Here's how the part is built. I have some questions about the finished solid (model axes, mm). Face numbers are marked on the shaded views. Round coordinates to 2 decimals unless told otherwise and drop trailing zeros. Loops run counter-clockwise (first coordinate to the right, second up) from the corner with the lowest first, then second, coordinate; pieces in that order, holes last. Notation, with made-up numbers: M 86,-21 L 104,-21 A14 ccw 104,4 Z; hole C 89.25,-8.75 d4. An arc over 180 degrees is marked long. Put each result on its own line as item: value. Start each with the question number.
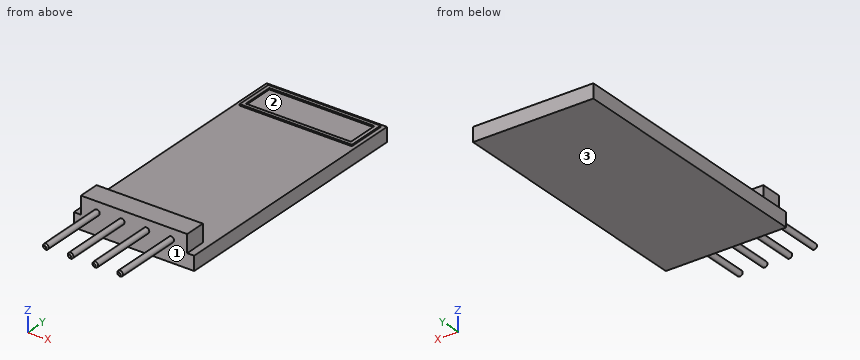
```python
from build123d import *

# Parameters (mm, degrees)
F0_W     = 17
F0_H     = 37
F1_DEPTH = 1
F2_W     = 15
F2_H     = 3
F3_DEPTH = 2.5
F4_R     = 0.4
F5_DEPTH = 10
F6_SIZE  = 0.2
F7_W     = 15.8485004902
F7_H     = 5.5060135201
F7_W_2   = 14.8485004902
F7_H_2   = 4.5060135201
F8_DEPTH = 0.2


with BuildPart() as f1:
    # F0 (on Top) → F1 (new body, symmetric)
    with BuildSketch(Plane.XY):
        Rectangle(F0_W, F0_H)
    extrude(amount=F1_DEPTH, both=True)

    # F2 (on face) → F3 (join)
    with BuildSketch(Plane.XY.offset(1)):
        with Locations((0, -17)):
            Rectangle(F2_W, F2_H)
    extrude(amount=F3_DEPTH)

    # F4 (on face) → F5 (join)
    with BuildSketch(Plane.XZ.offset(18.5)):
        with Locations((-5.25, 2.0477680955)):
            Circle(F4_R)
        with Locations((-1.75, 2.0477680955)):
            Circle(F4_R)
        with Locations((1.75, 2.0477680955)):
            Circle(F4_R)
        with Locations((5.25, 2.0477680955)):
            Circle(F4_R)
    extrude(amount=F5_DEPTH)

    # F6
    f6_edges = [f1.edges().sort_by_distance(p)[0] for p in [
        (-5.65, -28.5, 2.047768),
        (-2.15, -28.5, 2.047768),
        (1.35, -28.5, 2.047768),
        (4.85, -28.5, 2.047768),
    ]]
    chamfer(f6_edges, length=F6_SIZE)

    # F7 (on face) → F8 (join)
    with BuildSketch(Plane.XY.offset(1)):
        with Locations((0.0227517448, 15.2666731738)):
            Rectangle(F7_W, F7_H)
        with Locations((0.0227517448, 15.2666731738)):
            Rectangle(F7_W_2, F7_H_2, mode=Mode.SUBTRACT)
    extrude(amount=F8_DEPTH)


solid = f1.part
```
1) If we mould it in two halves opening along Y, with no side actions, what happens to the marked faces 1, 2 and 3? For each: pulls with the +Y half, pulls with the -Y half, needs draft (parallel to the pull), parting line crosses it, or undercut.
2) If I drill on probe 1 along Y at (x, z) = (2, 1.05); probe 2 along X at (y, z) = (16, 1.1); probe 3 along X at (y, z) = (-20.5, 1.9), over which ranges is the centre line in solid material (lowest first)? Write a range as from..to.
3) Suppose I cut it at B-B (z = 3). Write out the boundary of the cut face in (x, y), plus the area to 3 significant figures.
4) Suppose I cut it at A-A (x = 4). Write out the boundary of the cut face in (y, z), plus the area to 3 significant figures.
5) I'm going to push flat-ended pins straight in: P1, Ø1.4, axis at x = 2, y = 14.5, coming from the +Z side; P2, Ø10, axis at x = -6.5, y = 10, coming from the +Z side; P3, Ø1.3, axis at x = -3, z = 0.5, coming from the -Y side; P4, Ø8, axis at x = 5.5, y = -13, coming from the +Z side. Where does each tip first touch, or does it pass through?
6) Suppose I cut it at C-C (y = -2). Write out the boundary of the cut face in (x, z), plus the area to 3 significant figures.
Results are:
1. face 1: pulls with the -Y half
1. face 2: undercut
1. face 3: needs draft
2. probe 1: -18.5..-15.5, 12.51..13.01, 17.52..18.02
2. probe 2: -7.9..-7.4, 7.45..7.95
2. probe 3: -5.62..-4.88, -2.12..-1.38, 1.38..2.12, 4.88..5.62
3. outline: M -7.5,-18.5 L 7.5,-18.5 L 7.5,-15.5 L -7.5,-15.5 Z
3. area: 45.0 mm²
4. outline: M -18.5,-1 L 18.5,-1 L 18.5,1 L 18.02,1 L 18.02,1.2 L 17.52,1.2 L 17.52,1 L 13.01,1 L 13.01,1.2 L 12.51,1.2 L 12.51,1 L -15.5,1 L -15.5,3.5 L -18.5,3.5 Z
4. area: 81.7 mm²
5. P1: z = 1
5. P2: z = 1.2
5. P3: y = -18.5
5. P4: z = 3.5
6. outline: M -8.5,-1 L 8.5,-1 L 8.5,1 L -8.5,1 Z
6. area: 34.0 mm²
